Check sheet for the drawn part. Datum: minimum x, y, z corner. Units: mm. A direction names the side the tool comes from. Coordinates: 2 decimals unless noted, no trailing zeros. Write each loop counter-clockwise with the first axis right and the second up, starting at its lowest first coordinate (ties: lowest second). Pieces come first, ordered by that corner, then holes. Notation, with made-up numbers: (21, -31) -> (54, -31) arc R22 ccw to (54, 6) -> close; hole circle Ø7 at (-37, -28). An arc over 180 degrees is marked (long way). Write each question's results on one line, items separated by ' | '. Start each with the question number.
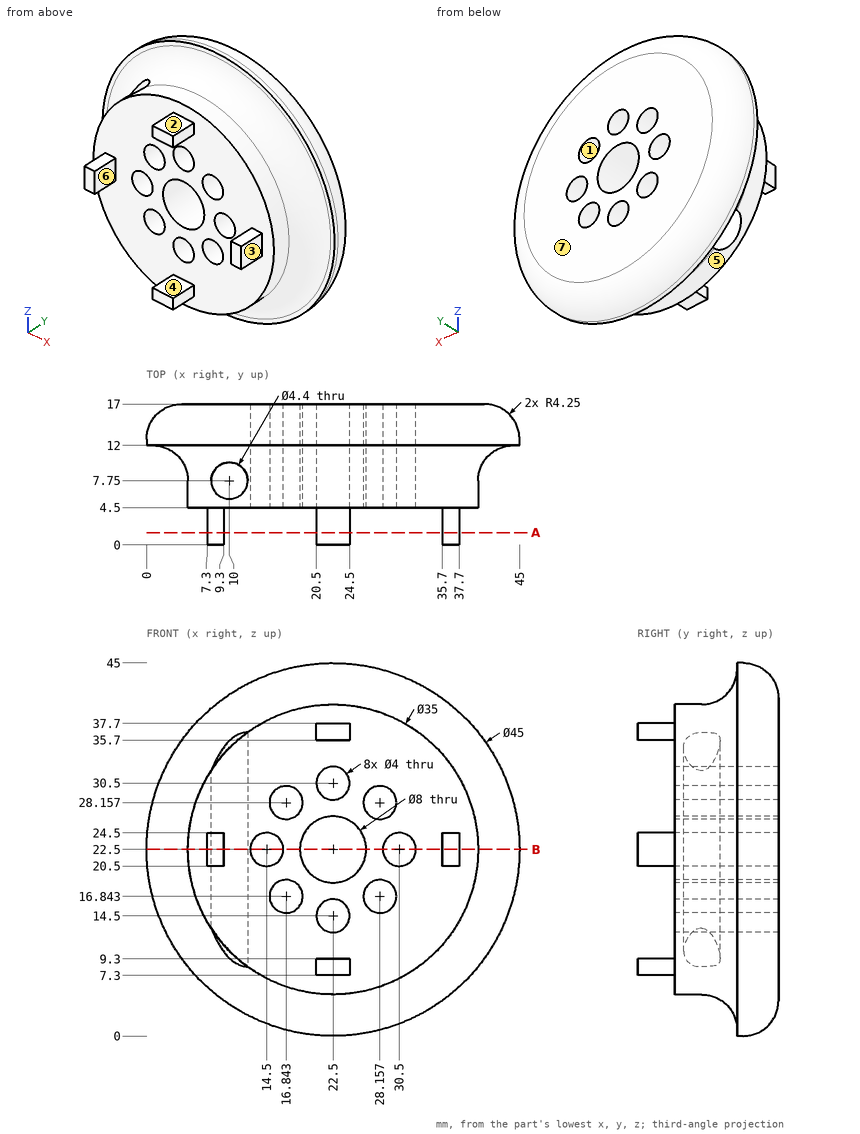
1. Sectioned sample at B-B on z = 22.5. State how many separate pieces and enclosed holes the cut face has, plus the area to 3 significant figures.
2. Depth check by flat-ended pin: pin 1 Ø4.5 at (x, z) = (14.5, 22.5) entering from -Y; pin 2 Ø1.6 at (y, z) = (2.5, 8) entering from +X; pin 3 Ø2.5 at (x, z) = (22.5, 30.5) entering from +Y; pin 4 Ø5 at (x, y) = (10, 7.75) entering from -Z. Enter the tip coordinate at first touch or a pass-through.
3. Material ranges on probe 1 along Y at (x, z) = (10, 26); probe 2 along X at (y, z) = (11.25, 27.5); probe 3 along X at (y, z) = (7.75, 17.5), recorded low to high. Write a range as from..to.
4. Sectioned sample at A-A on y = 1.5. Record the cut outline in (x, z).
5. Mould release check, pull along X, two halves, no side actions. Record for the marked faces 5, 6 and 7: +X half, -X half, draft (parallel to the pull), parting line (faces both ways), or undercut.
6. Tool access check on the marked faces 1, 2, 3 and 4. Record the directions out of +Z, -Z, +X, -X, +Y, -Y that give a thin tool (end or side, any length) a straight path to the whole face; none if there is none.
Computed values:
1) separate pieces: 4 | enclosed holes: 1 | area: 290 mm^2
2) pin 1: stops at y = 4.5 | pin 2: stops at x = 24.5 | pin 3: passes through | pin 4: stops at z = 8.14
3) probe 1: y = 4.5..5.55, 9.95..17 | probe 2: x = 3.82..14.95, 18.73..26.27, 30.05..41.18 | probe 3: x = 5.73..7.8, 12.2..14.95, 18.73..26.27, 30.05..39.27
4) outline: (7.3, 20.5) -> (9.3, 20.5) -> (9.3, 24.5) -> (7.3, 24.5) -> close; (20.5, 7.3) -> (24.5, 7.3) -> (24.5, 9.3) -> (20.5, 9.3) -> close; (20.5, 35.7) -> (24.5, 35.7) -> (24.5, 37.7) -> (20.5, 37.7) -> close; (35.7, 20.5) -> (37.7, 20.5) -> (37.7, 24.5) -> (35.7, 24.5) -> close
5) face 5: parting line | face 6: undercut | face 7: draft
6) face 1: +Y, -Y | face 2: +Z, +X, -X, -Y | face 3: +Z, -Z, +X, -Y | face 4: +X, -X, -Y
